from build123d import *

# Parameters (mm, degrees)
CHAMFER1_SIZE = 6


with BuildPart() as part:
    # Sketch1 → Revolve1 (revolve)
    with BuildSketch(Plane.XY, mode=Mode.PRIVATE) as revolve1_sk:
        Polygon((0, 0), (14.5, 0), (14.5, 10), (12.15, 10), (12.15, 12.35), (12.5, 12.35), (12.5, 34), (10.15, 34), (10.15, 36.35), (12.5, 36.35), (12.5, 78), (10.15, 78), (10.15, 80.35), (12.5, 80.35), (12.5, 122), (10.15, 122), (10.15, 124.35), (12.5, 124.35), (12.5, 166), (10.15, 166), (10.15, 168.35), (12.5, 168.35), (12.5, 210), (0, 210), align=None)
    revolve(revolve1_sk.sketch.rotate(Axis((0, 210, 0), (0, -1, 0)), 180), axis=Axis((0, 210, 0), (0, -1, 0)))

    # Chamfer1
    chamfer1_edges = [part.edges().sort_by_distance(p)[0] for p in [
        (12.5, 210, 0),
    ]]
    chamfer(chamfer1_edges, length=CHAMFER1_SIZE)


solid = part.part
Verification items for the finished model (mm, model axes). A direction names the side the tool comes from. Coordinates: 2 decimals unless noted, no trailing zeros. Loops run counter-clockwise (first coordinate to the right, second up) from the corner with the lowest first, then second, coordinate; pieces in that order, holes last. Notation, with made-up numbers: (69.5, 35) -> (123.5, 35) arc R6 ccw to (123.5, 43) -> close; hole circle Ø3 at (58.25, 58). An arc over 180 degrees is marked (long way). Answer as CSV lines item,"result".
1) Depth check by flat-ended pin: pin 1 (10 mm diameter, centred on x = -0.5, y = 96, fed in from -Z); pin 2 (10 mm diameter, centred on x = -11, z = 1.5, fed in from +Y); pin 3 (2 mm diameter, centred on x = -10, z = -2.5, fed in from +Y); pin 4 (10 mm diameter, centred on y = 40, z = 2.5, fed in from -X). Enter the tip coordinate at first touch or a pass-through.
Found:
pin 1,"stops at z = -12.5"
pin 2,"stops at y = 210"
pin 3,"stops at y = 207.19"
pin 4,"stops at x = -12.5"
2) Tool access check on faces 1 (the cylindrical face through (-11.59, 11.19, -3.65)), 2 (the cylindrical face through (-11.923, 23.327, -3.755)), 3 (the flat face through (0, 210, 0)). Record the directions out of +Z, -Z, +X, -X, +Y, -Y that give a thin tool (end or side, any length) a straight path to the whole face; none if there is none.
Found:
face 1,"none"
face 2,"+Y"
face 3,"+Z, -Z, +X, -X, +Y"
3) Cross-section at A-A, the plane y = 130. Record the cut outline in (x, z), then the cut area to 3 significant figures.
Found:
outline,"circle Ø25 at (0, 0)"
area,"491 mm2"
4) Release check for a two-part mould opening along Y. For faces 4 (the flat face through (1.9, 34, -10.2)), 5 (the conical face through (-6.5, 209.7, -2)), 6 (the cylindrical face through (-11.923, 57.467, -3.755)) record: +Y half, -Y half, draft (parallel to the pull), parting line (faces both ways), or undercut.
Found:
face 4,"undercut"
face 5,"+Y half"
face 6,"draft"
5) Thickness scan on L1, parallel to Z at x = -1, y = 111.5; L2, parallel to Y at x = -10.75, z = 6.25. Record the ranges inside material, lowest first. Write a range as from..to.
Found:
L1,"z = -12.46..12.46"
L2,"y = 0..10, 12.35..34, 36.35..78, 80.35..122, 124.35..166, 168.35..204.07"
